from build123d import *

# Parameters (mm, degrees)
FILLET_R    = 1
FILLET001_R = 1


with BuildPart() as part:
    # Sketch → Revolution (revolve)
    with BuildSketch(Plane.XY):
        Polygon((0, 0), (-36.5, 0), (-40, 68), (-42, 68), (-38.397059, -2), (0, -2), align=None)
    revolve(axis=Axis((0, 0, 0), (0, 1, 0)))

    # Fillet
    fillet_edges = [part.edges().sort_by_distance(p)[0] for p in [
        (38.397059, -2, 0),
    ]]
    fillet(fillet_edges, radius=FILLET_R)

    # Fillet001
    fillet001_edges = [part.edges().sort_by_distance(p)[0] for p in [
        (36.5, 0, 0),
    ]]
    fillet(fillet001_edges, radius=FILLET001_R)


with BuildPart() as part_1:
    # Body001 placement: moved
    add(part.part.moved(Location((15.758551, 56.807331, -3.324877))))


solid = part_1.part
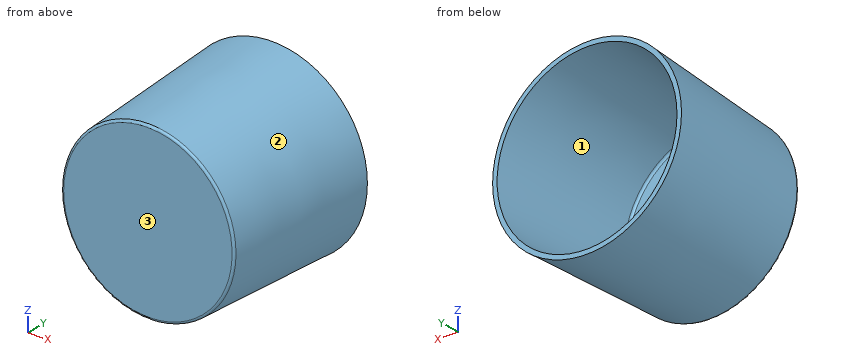
The model under review builds one solid part; all positions refer to its coordinate system, in mm. Face numbers are marked on the shaded views. Coordinates: 2 decimals unless noted, no trailing zeros. Order: outer loops, then holes, each group sorted by start corner. A loop starts at its lowest first (then second) coordinate and runs counter-clockwise, first axis right, second up. Notation, with made-up numbers: (-12.75, 88.5) -> (27.25, 88.5) arc R7 cw to (27.25, 99.5) -> close; hole circle Ø1 at (4, -2). An arc over 180 degrees is marked (long way). Answer in a Markdown table with one row per item.
(1) Insertion check: pin 1 (1 mm diameter, centred on y = 100.5, z = 4, fed in from -X); pin 2 (1.5 mm diameter, centred on x = 32.5, y = 107.5, fed in from -Z); pin 3 (2 mm diameter, centred on y = 106, z = 24, fed in from +X). Each pin has a flat end and moves straight along its axis. Give the tip position at first contact, or say it passes through.
Answers:
| item | result |
|---|---|
| pin 1 | x = -24.42 |
| pin 2 | z = -41.2 |
| pin 3 | x = 47.24 |
(2) Consider section B-B (y = 114.5). Write out the cut boundary in (x, z), plus the area to 3 significant figures.
Answers:
| item | result |
|---|---|
| outline | circle Ø82.94 at (15.76, -3.32); hole circle Ø78.94 at (15.76, -3.32) |
| area | 509 mm² |
(3) The part is to be moulded in two halves that separate along Z. For the marked faces 1, 2 and 3, say which applies: +Z half, -Z half, draft (parallel to the pull), parting line (faces both ways), or undercut.
Answers:
| item | result |
|---|---|
| face 1 | undercut |
| face 2 | parting line |
| face 3 | draft |
(4) Wall thickness on line 1 along Y through (x, z) = (47, 4); line 2 along Z through (x, y) = (22, 62); line 3 along Z through (x, y) = (42.5, 81.5): over which ranges is each line inside the solid? List them lowest first.
Answers:
| item | result |
|---|---|
| line 1 | 54.81 to 56.81 |
| line 2 | -41.59 to -39.56, 32.91 to 34.94 |
| line 3 | -32.76 to -30, 23.35 to 26.11 |
(5) Consider section A-A (y = 105). Write out the cut boundary in (x, z), plus the area to 3 significant figures.
Answers:
| item | result |
|---|---|
| outline | circle Ø81.96 at (15.76, -3.32); hole circle Ø77.96 at (15.76, -3.32) |
| area | 502 mm² |
